Geometry: final body of the model. Coordinates: model frame, mm. A direction names the side the tool comes from. Coordinates: 2 decimals unless noted, no trailing zeros. Write each loop counter-clockwise with the first axis right and the second up, starting at its lowest first coordinate (ties: lowest second). Pieces come first, ordered by that corner, then holes. Notation, with made-up numbers: (59.25, -5.5) -> (109.25, -5.5) arc R25 ccw to (109.25, 17.5) -> close; hole circle Ø1 at (34.25, 7.5). An arc over 180 degrees is marked (long way). Answer as a JSON object with one key per item and string values. Group by question number.
```python
from build123d import *

# Parameters (mm, degrees)
F0_W      = 33.528
F0_H      = 5.08
F1_DEPTH  = 16.383
F2_W      = 33.528
F2_H      = 5.969
F3_DEPTH  = 11.43
F4_SIZE   = 11.43
F5_R      = 2.159
F6_DEPTH  = 25.4
F7_W      = 3.048
F7_H      = 2.54
F8_DEPTH  = 2.54
F9_W      = 4.191
F9_H      = 2.54
F10_DEPTH = 2.4638
F11_R     = 5.08


with BuildPart() as f1:
    # F0 (on Top) → F1 (new body)
    with BuildSketch(Plane.XY):
        with Locations((4.3383603916, 8.4559087365)):
            Rectangle(F0_W, F0_H)
    extrude(amount=F1_DEPTH)

    # F2 (on face) → F3 (join)
    with BuildSketch(Plane(origin=(0, 10.9959087365, 0), x_dir=(-1, 0, 0), z_dir=(0, 1, 0))):
        with Locations((-4.3383603916, 8.1915)):
            Rectangle(F2_W, F2_H)
    extrude(amount=F3_DEPTH)

    # F4
    f4_edges = [f1.edges().sort_by_distance(p)[0] for p in [
        (-12.42564, 22.425909, 8.1915),
        (21.10236, 22.425909, 8.1915),
    ]]
    chamfer(f4_edges, length=F4_SIZE)

    # F5 (on face) → F6 (cut)
    with BuildSketch(Plane(origin=(0, 0, 5.207), x_dir=(1, 0, 0), z_dir=(0, 0, -1))):
        with Locations((4.3383603916, -16.0759087365)):
            Circle(F5_R)
    extrude(amount=-F6_DEPTH, mode=Mode.SUBTRACT)

    # F7 (on face) → F8 (join)
    with BuildSketch(Plane.XZ.offset(-5.9159087365)):
        with Locations((17.0383603916, 12.573)):
            Rectangle(F7_W, F7_H)
    extrude(amount=F8_DEPTH)

    # F9 (on face) → F10 (join)
    with BuildSketch(Plane.XZ.offset(-5.9159087365)):
        with Locations((17.0383603916, 8.128)):
            Rectangle(F9_W, F9_H)
    extrude(amount=F10_DEPTH)

    # F11
    f11_edges = [f1.edges().sort_by_distance(p)[0] for p in [
        (-0.99564, 22.425909, 8.1915),
        (9.67236, 22.425909, 8.1915),
    ]]
    fillet(f11_edges, radius=F11_R)


solid = f1.part
```
Item 1: Set-up query: faces 1 (the flat face through (17, 5, 6.858)), 2 (the flat face through (4, 10.996, 14)), 3 (the flat face through (15.514, 5, 13)). Return all of +Z, -Z, +X, -X, +Y, -Y with unobstructed straight access to the full face (end or side cutting, diameter ignored); none if empty.
Item 2: Mould query, pull axis Z, two halves, no side actions, for faces 4 (the flat face through (17, 5, 11.303)), 5 (the flat face through (17, 5, 13.843)), 6 (the flat face through (17, 5, 9.398)), 7 (the flat face through (19.134, 5, 8)). Classes: +Z half, -Z half, draft (parallel to the pull), parting line (faces both ways), or undercut.
Item 3: Section C-C on x = -2. Output: boundary loops of the cut face in (y, z).
Item 4: Section B-B on z = 10. Output: boundary loops of the cut face in (x, y).
Item 5: Contact query for flat-ended pins moving along their axis: pin 1 (8 mm diameter, centred on x = 16, y = 15.5, fed in from -Z); pin 2 (0.7 mm diameter, centred on y = 4.5, z = 8, fed in from +X); pin 3 (1.3 mm diameter, centred on x = 17.5, y = 4.5, fed in from -Z). Output: stop coordinate, or through.
Item 6: Ray query, L1, parallel to Y at x = -4, z = 13.75; L2, parallel to Z at x = 3, y = 19.25; L3, parallel to X at y = 5.75, z = 11.5. Return the intervals inside material, ascending. Write a range as [from, to].
Item 7: Section D-D on y = 12.5. Output: boundary loops of the cut face in (x, z), then the cut area to 3 significant figures.
Item 8: Section A-A on z = 12.25. Output: boundary loops of the cut face in (x, y), then the cut area to 3 significant figures.
Answer sheet:
{
 "1": {"face 1": "-Z, +X, -X, -Y", "face 2": "+Z, +X, -X, +Y", "face 3": "+Z, -X, -Y"},
 "2": {"face 4": "undercut", "face 5": "+Z half", "face 6": "undercut", "face 7": "draft"},
 "3": {"outline": "(5.92, 0) -> (11, 0) -> (11, 5.21) -> (21.36, 5.21) -> (21.36, 11.18) -> (11, 11.18) -> (11, 16.38) -> (5.92, 16.38) -> close"},
 "4": {"outline": "(-12.43, 5.92) -> (21.1, 5.92) -> (21.1, 11) -> (11.16, 20.94) arc R5.08 ccw to (7.57, 22.43) -> (1.11, 22.43) arc R5.08 ccw to (-2.48, 20.94) -> (-12.43, 11) -> close; hole circle Ø4.32 at (4.34, 16.08)"},
 "5": {"pin 1": "stops at z = 5.21", "pin 2": "stops at x = 19.13", "pin 3": "stops at z = 6.86"},
 "6": {"L1": "y = [5.92, 11]", "L2": "z = [5.21, 11.18]", "L3": "x = [15.51, 18.56]"},
 "7": {"outline": "(-10.92, 5.21) -> (19.6, 5.21) -> (19.6, 11.18) -> (-10.92, 11.18) -> close", "area": "182 mm^2"},
 "8": {"outline": "(-12.43, 5.92) -> (15.51, 5.92) -> (15.51, 3.38) -> (18.56, 3.38) -> (18.56, 5.92) -> (21.1, 5.92) -> (21.1, 11) -> (-12.43, 11) -> close", "area": "178 mm^2"}
}
